from build123d import *

# Parameters (mm, degrees)
SKETCH1_W               = 172.72
SKETCH1_H               = 38.1
BOSS_EXTRUDE1_DEPTH     = 12.7
SKETCH2_W               = 12.7
SKETCH2_H               = 38.1
BOSS_EXTRUDE2_DEPTH     = 38.1
SKETCH3_R               = 19.05
BOSS_EXTRUDE3_DEPTH     = 508
BOSS_EXTRUDE5_DEPTH     = 19.05
FILLET3_R               = 19.05
CUT_EXTRUDE1_DEPTH      = 638.105779031
CUT_EXTRUDE1_DEPTH_BACK = 638.105779031
SKETCH5_R               = 5.08


with BuildPart() as part:
    # Sketch1 → Boss-Extrude1 (new body)
    with BuildSketch(Plane.XY):
        Rectangle(SKETCH1_W, SKETCH1_H)
    extrude(amount=BOSS_EXTRUDE1_DEPTH)

    # Sketch2 → Boss-Extrude2 (add)
    with BuildSketch(Plane.XY.offset(12.7)):
        with Locations((-80.01, 0)):
            Rectangle(SKETCH2_W, SKETCH2_H)
        with Locations((80.01, 0)):
            Rectangle(SKETCH2_W, SKETCH2_H)
    extrude(amount=BOSS_EXTRUDE2_DEPTH)

    # Sketch3 → Boss-Extrude3 (add)
    with BuildSketch(Plane(origin=(0, 0, 0), x_dir=(-1, 0, 0), z_dir=(0, 0, -1))):
        with Locations(Location((-67.31, 0, 0), (0, 0, 180))):
            Circle(SKETCH3_R)
        with Locations((67.31, 0)):
            Circle(SKETCH3_R)
    extrude(amount=BOSS_EXTRUDE3_DEPTH)

    # Sketch4 → Boss-Extrude5 (add, symmetric)
    with BuildSketch(Plane(origin=(0, 0, 0), x_dir=(1, 0, 0), z_dir=(0, 1, 0))):
        Polygon((-86.36, 616.388246785), (86.36, 616.388246785), (86.36, 573.352506856), (86.36, 508), (48.26, 508), (48.26, 573.352506856), (-48.26, 573.352506856), (-48.26, 508), (-86.36, 508), (-86.36, 573.352506856), align=None)
    extrude(amount=BOSS_EXTRUDE5_DEPTH, both=True)

    # Fillet3
    fillet3_edges = [part.edges().sort_by_distance(p)[0] for p in [
        (86.36, -19.05, -562.194123393),
        (0, -19.05, -616.388246785),
        (86.36, 0, -616.388246785),
        (-86.36, -19.05, -562.194123393),
        (-86.36, 0, -616.388246785),
        (-48.26, -19.05, -540.676253428),
        (0, -19.05, -573.352506856),
        (-48.26, 0, -573.352506856),
        (48.26, -19.05, -540.676253428),
        (48.26, 0, -573.352506856),
        (86.36, 19.05, -562.194123393),
        (0, 19.05, -616.388246785),
        (-86.36, 19.05, -562.194123393),
        (-48.26, 19.05, -540.676253428),
        (0, 19.05, -573.352506856),
        (48.26, 19.05, -540.676253428),
    ]]
    fillet(fillet3_edges, radius=FILLET3_R - 0.0001)  # a hair under: the kernel refuses the full size

    # Sketch5 → Cut-Extrude1 (cut, two sides: drawn at the far end of the back side and taken through both)
    with BuildSketch(Plane(origin=(-73.66, 0, 0), x_dir=(0, 0, -1), z_dir=(1, 0, 0)).offset(-CUT_EXTRUDE1_DEPTH_BACK)):
        with Locations((-31.75, 0)):
            Circle(SKETCH5_R)
    extrude(amount=CUT_EXTRUDE1_DEPTH + CUT_EXTRUDE1_DEPTH_BACK, mode=Mode.SUBTRACT)


solid = part.part
Build history of the part. All positions in model axes, mm. A direction names the side the tool comes from. Coordinates: 2 decimals unless noted, no trailing zeros. Write each loop counter-clockwise with the first axis right and the second up, starting at its lowest first coordinate (ties: lowest second). Pieces come first, ordered by that corner, then holes. Notation, with made-up numbers: (56.5, -28) -> (89.5, -28) arc R27 cw to (89.5, 5) -> close; hole circle Ø9 at (31, -0.75). An arc over 180 degrees is marked (long way). Use CSV: the item, a comma, the result in double quotes. Start each with the question number.
Q1. 3-axis set-ups, long thin cutter, end or side, ignore diameter. For faces 5 (the cylindrical face through (-0.409, -13.618, -579.081)), 6 (the flat face through (82, -15, 0)), 7 (the flat face through (-73.66, 4, 27)), 8 (the cylindrical face through (-0.409, 13.618, -579.081)): which of +Z, -Z, +X, -X, +Y, -Y reach the whole face in a straight line?
Q2. Drill centre lines: probe 1 along X at (y, z) = (0.5, -279.5); probe 2 along Y at (x, z) = (-83, 31); probe 3 along X at (y, z) = (10, -568). Where is each one in solid material? Low to high.
Q3. Flat gauge pins, fed straight in: pin 1 Ø5.5 at (x, y) = (74.5, 10) entering from -Z; pin 2 Ø9.5 at (x, y) = (55, 7.5) entering from +Z; pin 3 Ø10 at (y, z) = (-14.5, -113.5) entering from -X; pin 4 Ø10 at (x, y) = (-65.5, 3) entering from -Z. Where does each tip first touch, or does it go through?
Q4. Cut at B-B, the plane z = -174. List the corners of the cut face in (x, y).
Q5. Pull direction Z, two halves, no side cores. Call faces 1 (the cylindrical face through (-84.907, -7.296, -250.444)), 2 (the flat face through (0, -19.05, -593)), 3 (the cylindrical face through (0.94, -13.32, -610.96)), 4 (the flat face through (-80, 0, 50.8)): released by +Z, released by -Z, zero draft, split by the parting line, or undercut.
Checked values:
1,face 5,"-Y"
1,face 6,"-Z, +X, -Y"
1,face 7,"+Z, +Y, -Y"
1,face 8,"+Y"
2,probe 1,"x = -86.35 to -48.27, 48.27 to 86.35"
2,probe 2,"y = -19.05 to -5.02, 5.02 to 19.05"
2,probe 3,"x = -83.52 to -46.28, 46.28 to 83.52"
3,pin 1,"stops at z = -613.81"
3,pin 2,"stops at z = 12.7"
3,pin 3,"stops at x = -83.82"
3,pin 4,"stops at z = -616.39"
4,outline,"circle Ø38.1 at (-67.31, 0); circle Ø38.1 at (67.31, 0)"
5,face 1,"undercut"
5,face 2,"zero draft"
5,face 3,"released by -Z"
5,face 4,"released by +Z"
